```python
from build123d import *

# Parameters (mm, degrees)
F1_DEPTH = 5
F2_R     = 3
F2_R_2   = 3.175833
F3_DEPTH = 25
F4_R     = 3
F5_DEPTH = 25
F6_R     = 2.5
F7_DEPTH = 10


with BuildPart() as f1:
    # F0 (on Top) → F1 (new body, symmetric)
    with BuildSketch(Plane.XY):
        Polygon((335, -25), (335, 25), (185, 25), (-185, 25), (-335, 25), (-335, -25), align=None)
        Polygon((185, 25), (335, 25), (335, 125), (305, 125), align=None)
        Polygon((-335, 25), (-185, 25), (-305, 125), (-335, 125), align=None)
    extrude(amount=F1_DEPTH, both=True)

    # F2 (on face) → F3 (cut)
    with BuildSketch(Plane.YZ.offset(335)):
        with Locations((26, 0)):
            Circle(F2_R)
        with Locations((-14, 0)):
            Circle(F2_R)
        with Locations((74, 0)):
            Circle(F2_R_2)
        with Locations((114, 0)):
            Circle(F2_R)
    extrude(amount=-F3_DEPTH, mode=Mode.SUBTRACT)

    # F4 (on face) → F5 (cut)
    with BuildSketch(Plane(origin=(-335, 0, 0), x_dir=(0, -1, 0), z_dir=(-1, 0, 0))):
        with Locations((14, 0)):
            Circle(F4_R)
        with Locations((-26, 0)):
            Circle(F4_R)
        with Locations((-74, 0)):
            Circle(F4_R)
        with Locations((-114, 0)):
            Circle(F4_R)
    extrude(amount=-F5_DEPTH, mode=Mode.SUBTRACT)

    # F6 (on face) → F7 (cut)
    with BuildSketch(Plane.XY.offset(5)):
        with Locations((-20, 12)):
            Circle(F6_R)
        with Locations((20, 12)):
            Circle(F6_R)
        with Locations((20, -12)):
            Circle(F6_R)
        with Locations((-20, -12)):
            Circle(F6_R)
    extrude(amount=-F7_DEPTH, mode=Mode.SUBTRACT)


solid = f1.part
```
Geometry: final body of the model. Coordinates: model frame, mm. A direction names the side the tool comes from. Round coordinates to 2 decimals unless told otherwise and drop trailing zeros. Order: outer loops, then holes, each group sorted by start corner. A loop starts at its lowest first (then second) coordinate and runs counter-clockwise, first axis right, second up. Notation, with made-up numbers: (70, 37.25) -> (127, 37.25) arc R19 cw to (127, 44.25) -> close; hole circle Ø1 at (66.5, 58). An arc over 180 degrees is marked (long way). Write each question's results on one line, items separated by ' | '.
Q1. Pin query (flat end, axial travel): pin 1 Ø5 at (x, z) = (-54, 3) entering from +Y; pin 2 Ø5 at (y, z) = (74, 0) entering from -X; pin 3 Ø3 at (y, z) = (26.5, -1) entering from +X. Return the tip coordinate at first contact, or that it passes through.
Response values:
pin 1: y = 25 | pin 2: x = -310 | pin 3: x = 310
Q2. Ray query, line 1 along Y through (x, z) = (-20, -1); line 2 along Z through (x, y) = (-319, 26); line 3 along Z through (x, y) = (329, 74). Return the intervals inside material, ascending.
Response values:
line 1: -25 to -14.5, -9.5 to 9.5, 14.5 to 25 | line 2: -5 to -3, 3 to 5 | line 3: -5 to -3.18, 3.18 to 5
Q3. Access query for faces 1 (the face through (-5, 18, 5)), 2 (the face through (245.84, 75.7, 0.07)). Directions: +Z, -Z, +X, -X, +Y, -Y. A direction counts if a zero-diameter tool reaches every point of the face in a straight line with its end or side. Return the directions, or none.
Response values:
face 1: +Z, +X, -X, +Y, -Y | face 2: +Z, -Z, +Y
Q4. Section query C-C (x = 74). Output: boundary loops of the cut face in (y, z), and give its area (3 significant figures).
Response values:
outline: (-25, -5) -> (25, -5) -> (25, 5) -> (-25, 5) -> close | area: 500 mm²
Q5. Section query B-B (y = 84). Output: boundary loops of the cut face in (x, z), and give its area (3 significant figures).
Response values:
outline: (-335, -5) -> (-255.8, -5) -> (-255.8, 5) -> (-335, 5) -> close; (255.8, -5) -> (335, -5) -> (335, 5) -> (255.8, 5) -> close | area: 1,580 mm²
Q6. Section query A-A (y = 51). Output: boundary loops of the cut face in (x, z), and give its area (3 significant figures).
Response values:
outline: (-335, -5) -> (-216.2, -5) -> (-216.2, 5) -> (-335, 5) -> close; (216.2, -5) -> (335, -5) -> (335, 5) -> (216.2, 5) -> close | area: 2,380 mm²
Q7. Pull-direction query (X, two-part tool) for faces 3 (the face through (-5, 18, -5)), 4 (the face through (-244.16, 74.3, 0.07)); classes: released by +X, released by -X, zero draft, split by the parting line, or undercut.
Response values:
face 3: zero draft | face 4: undercut
